```python
from build123d import *

# Parameters (mm, degrees)
F0_W     = 10
F0_H     = 11
F1_DEPTH = 12
F3_DEPTH = 5.67
F5_DEPTH = 1.6
F6_DEPTH = 9
F7_SIZE  = 1
F8_W     = 0.64
F8_H     = 0.36
F9_DEPTH = 4
F10_SIZE = 0.1


with BuildPart() as f1:
    # F0 (on Top) → F1 (new body)
    with BuildSketch(Plane.XY):
        Rectangle(F0_W, F0_H)
    extrude(amount=F1_DEPTH)

    # F2 (on face) → F3 (join)
    with BuildSketch(Plane.XY.offset(12)):
        with BuildLine():
            ThreePointArc((1.7748239349, -2.4), (2.9660075336, -1.1621670526), (3.4, 0.5))
            ThreePointArc((3.4, 0.5), (2.9660075336, 2.1621670526), (1.7748239349, 3.4))
            Line((1.7748239349, 3.4), (-1.7748239349, 3.4))
            ThreePointArc((-1.7748239349, 3.4), (-3.4, 0.5), (-1.7748239349, -2.4))
            Line((-1.7748239349, -2.4), (1.7748239349, -2.4))
        make_face()
    extrude(amount=F3_DEPTH)

    # F4 (on face) → F5 (join)
    with BuildSketch(Plane.XY.offset(17.67)):
        with BuildLine():
            ThreePointArc((1.4997051578, -2.0982464163), (2.5979910963, -1.0001474139), (3, 0.5))
            ThreePointArc((3, 0.5), (2.5807277905, 2.0296548863), (1.4401039525, 3.1317485834))
            Line((1.4401039525, 3.1317485834), (1.4997051578, -2.0982464163))
        make_face()
    extrude(amount=F5_DEPTH)

    # F4 (on face) → F6 (join)
    with BuildSketch(Plane.XY.offset(17.67)):
        with BuildLine():
            Line((1.4997051578, -2.0982464163), (1.4401039525, 3.1317485834))
            ThreePointArc((1.4401039525, 3.1317485834), (1.1122261333, 3.2862076427), (0.7681145748, 3.4))
            Line((0.7681145748, 3.4), (-0.7681145748, 3.4))
            ThreePointArc((-0.7681145748, 3.4), (-3, 0.5), (-0.7681145748, -2.4))
            Line((-0.7681145748, -2.4), (0.7681145748, -2.4))
            ThreePointArc((0.7681145748, -2.4), (1.143903576, -2.2733525937), (1.4997051578, -2.0982464163))
        make_face()
        with BuildLine():
            ThreePointArc((-0.7681145748, -2.4), (0, -2.5), (0.7681145748, -2.4))
            Line((0.7681145748, -2.4), (-0.7681145748, -2.4))
        make_face()
        with BuildLine():
            Line((-0.7681145748, 3.4), (0.7681145748, 3.4))
            ThreePointArc((0.7681145748, 3.4), (0, 3.5), (-0.7681145748, 3.4))
        make_face()
    extrude(amount=F6_DEPTH)

    # F7
    f7_edges = [f1.edges().sort_by_distance(p)[0] for p in [
        (-2.999805, 0.465814, 26.67),
    ]]
    chamfer(f7_edges, length=F7_SIZE)

    # F8 (on face) → F9 (join)
    with BuildSketch(Plane.XZ.offset(5.5)):
        with Locations((-4.68, 6.6)):
            Rectangle(F8_W, F8_H)
        with Locations((-2.34, 6.6)):
            Rectangle(F8_W, F8_H)
        with Locations((0, 6.6)):
            Rectangle(F8_W, F8_H)
        with Locations((4.68, 1.6)):
            Rectangle(F8_W, F8_H)
        with Locations((2.34, 1.6)):
            Rectangle(F8_W, F8_H)
        with Locations((0, 1.6)):
            Rectangle(F8_W, F8_H)
        with Locations((-2.34, 1.6)):
            Rectangle(F8_W, F8_H)
        with Locations((-4.68, 1.6)):
            Rectangle(F8_W, F8_H)
        with Locations((2.34, 6.6)):
            Rectangle(F8_W, F8_H)
        with Locations((4.68, 6.6)):
            Rectangle(F8_W, F8_H)
    extrude(amount=F9_DEPTH)

    # F10
    f10_edges = [f1.edges().sort_by_distance(p)[0] for p in [
        (-5, -9.5, 6.6),
        (-4.68, -9.5, 6.42),
        (-4.36, -9.5, 6.6),
        (-4.68, -9.5, 6.78),
        (-2.66, -9.5, 6.6),
        (-2.34, -9.5, 6.42),
        (-2.02, -9.5, 6.6),
        (-2.34, -9.5, 6.78),
        (-0.32, -9.5, 6.6),
        (0, -9.5, 6.42),
        (0.32, -9.5, 6.6),
        (0, -9.5, 6.78),
        (2.02, -9.5, 6.6),
        (2.34, -9.5, 6.42),
        (2.66, -9.5, 6.6),
        (2.34, -9.5, 6.78),
        (4.68, -9.5, 6.42),
        (5, -9.5, 6.6),
        (4.68, -9.5, 6.78),
        (4.36, -9.5, 6.6),
        (4.68, -9.5, 1.42),
        (5, -9.5, 1.6),
        (4.68, -9.5, 1.78),
        (4.36, -9.5, 1.6),
        (2.02, -9.5, 1.6),
        (2.34, -9.5, 1.42),
        (2.66, -9.5, 1.6),
        (2.34, -9.5, 1.78),
        (-0.32, -9.5, 1.6),
        (0, -9.5, 1.42),
        (0.32, -9.5, 1.6),
        (0, -9.5, 1.78),
        (-2.66, -9.5, 1.6),
        (-2.34, -9.5, 1.42),
        (-2.02, -9.5, 1.6),
        (-2.34, -9.5, 1.78),
        (-5, -9.5, 1.6),
        (-4.68, -9.5, 1.42),
        (-4.36, -9.5, 1.6),
        (-4.68, -9.5, 1.78),
    ]]
    chamfer(f10_edges, length=F10_SIZE)


solid = f1.part
```
The listing builds one solid part. Answer for the finished solid, in the listing's coordinates (mm). A direction names the side the tool comes from. Coordinates: 2 decimals unless noted, no trailing zeros. Write each loop counter-clockwise with the first axis right and the second up, starting at its lowest first coordinate (ties: lowest second). Pieces come first, ordered by that corner, then holes. Notation, with made-up numbers: (32, 45) - (41, 45) arc R23 ccw to (41, 72) - close; hole circle Ø5 at (28, -28.5). An arc over 180 degrees is marked (long way). One line per item, written item: value.
1) Find section B-B (y = -8). Count the separate pieces of the cut face and the enclosed holes in it, and give its area (3 significant figures).
Geometry check:
separate pieces: 10
enclosed holes: 0
area: 2.30 mm2
2) Find section D-D (z = 15). Give the vertices of the cut face in (x, y).
Geometry check:
outline: (-1.77, -2.4) - (1.77, -2.4) arc R3.4 ccw to (1.77, 3.4) - (-1.77, 3.4) arc R3.4 ccw to start
3) Each of these flat-tipped pins is pushed along its axis until it touches: pin 1 Ø3 at (x, z) = (-0.5, 14.5) entering from -Y; pin 2 Ø2 at (y, z) = (0.5, 22.5) entering from +X; pin 3 Ø0.5 at (x, y) = (-2.5, -7.5) entering from -Z. Where does it stop, or does it pass through?
Geometry check:
pin 1: stops at y = -2.4
pin 2: stops at x = 1.48
pin 3: stops at z = 1.42
4) Find section A-A (z = 22.75). Give the vertices of the cut face in (x, y), and give its area (3 significant figures).
Geometry check:
outline: (1.44, 3.13) arc R3 ccw (long way) to (1.5, -2.1) - close
area: 22.6 mm2
5) A tool of negligible diameter and unlimited length cuts with its end or side. For faces 4 (the flat face through (0, -2.4, 15)), 5 (the flat face through (0, 0, 0)), 6 (the cylindrical face through (-3.4, 0.5, 14.8)), from which of +Z, -Z, +X, -X, +Y, -Y can it reach the whole face along a straight path? Write none if from no direction.
Geometry check:
face 4: +X, -X, -Y
face 5: -Z, +X, -X, +Y, -Y
face 6: +Z, -X
6) Find section C-C (x = -4). Give the vertices of the cut face in (y, z), and give its area (3 significant figures).
Geometry check:
outline: (-5.5, 0) - (5.5, 0) - (5.5, 12) - (-5.5, 12) - close
area: 132 mm2
7) Consider line 1 along Z through (x, y) = (-0.25, -7); line 2 along Y through (x, z) = (3.75, 6.5); line 3 along Z through (x, y) = (3.5, -3.75). Determine where each line is inside the solid, lowest interval first. Write a range as from..to.
Geometry check:
line 1: z = 1.42..1.78, 6.42..6.78
line 2: y = -5.5..5.5
line 3: z = 0..12
8) For a pull along Z with two mould halves and no side action, classify faces 1 (the flat face through (0, 3.4, 15)), 2 (the flat face through (3.2, 0.7, 17.67)), 3 (the flat face through (0, 5.5, 6)) as pulls with the +Z half, pulls with the -Z half, needs draft (parallel to the pull), parting line crosses it, or undercut.
Geometry check:
face 1: undercut
face 2: pulls with the +Z half
face 3: needs draft
